```python
from build123d import *

# Parameters (mm, degrees)
SKETCH1_R                = 19.5
OUTERDIAMETERSTOCK_DEPTH = 115
SCREWONBASE_START        = -115
SCREWONBASE_DEPTH        = 5
INNERDIAMETER_START      = -3
SKETCH2_R                = 16
INNERDIAMETER_DEPTH      = 113
SKETCH3_R                = 10
HOLE_DEPTH               = 116
CUT_EXTRUDE3_REACH       = 117
SKETCH5_R                = 1.25
CHAMFER1_SIZE            = 1.5
WIRESLOT_START           = -115
SKETCH6_W                = 50
SKETCH6_H                = 20
WIRESLOT_DEPTH           = 10
MOUNTING_START           = -115
SKETCH7_R                = 2.5
MOUNTING_HOLES_DEPTH     = 5


with BuildPart() as part:
    # Sketch1 → OuterDiameterStock (new body)
    with BuildSketch(Plane(origin=(0, 0, 0), x_dir=(1, 0, 0), z_dir=(0, 1, 0))):
        Circle(SKETCH1_R)
    extrude(amount=-OUTERDIAMETERSTOCK_DEPTH)

    # Sketch4 → ScrewOnBase (add)
    with BuildSketch(Plane(origin=(0, 0, 0), x_dir=(1, 0, 0), z_dir=(0, 1, 0)).offset(SCREWONBASE_START)):
        with BuildLine():
            Line((0, 22.5), (50, 22.5))
            Line((50, 22.5), (50, -22.5))
            Line((50, -22.5), (0, -22.5))
            ThreePointArc((0, -22.5), (-22.5, 0), (0, 22.5))
        make_face()
    extrude(amount=SCREWONBASE_DEPTH)

    # Sketch2 → InnerDiameter (cut, through all)
    with BuildSketch(Plane(origin=(0, 0, 0), x_dir=(1, 0, 0), z_dir=(0, 1, 0)).offset(INNERDIAMETER_START)):
        Circle(SKETCH2_R)
    extrude(amount=-INNERDIAMETER_DEPTH, mode=Mode.SUBTRACT)

    # Sketch3 → Hole (cut, through all)
    with BuildSketch(Plane(origin=(0, 0, 0), x_dir=(1, 0, 0), z_dir=(0, 1, 0))):
        Circle(SKETCH3_R)
    extrude(amount=-HOLE_DEPTH, mode=Mode.SUBTRACT)

    # Sketch5 → Cut-Extrude3 (cut, up to next)
    with BuildSketch(Plane(origin=(0, 0, 0), x_dir=(1, 0, 0), z_dir=(0, 1, 0)), mode=Mode.PRIVATE) as cut_extrude3_sk1:
        with Locations((0, 13)):
            Circle(SKETCH5_R)
    cut_extrude3_tool1 = extrude(cut_extrude3_sk1.sketch, amount=-CUT_EXTRUDE3_REACH, mode=Mode.PRIVATE) & part.part
    add(cut_extrude3_tool1.solids().sort_by_distance((0, 0, -13))[0], mode=Mode.SUBTRACT)
    # Sketch5 → Cut-Extrude3 (cut, up to next)
    with BuildSketch(Plane(origin=(0, 0, 0), x_dir=(1, 0, 0), z_dir=(0, 1, 0)), mode=Mode.PRIVATE) as cut_extrude3_sk2:
        with Locations((13, 0)):
            Circle(SKETCH5_R)
    cut_extrude3_tool2 = extrude(cut_extrude3_sk2.sketch, amount=-CUT_EXTRUDE3_REACH, mode=Mode.PRIVATE) & part.part
    add(cut_extrude3_tool2.solids().sort_by_distance((13, 0, 0))[0], mode=Mode.SUBTRACT)
    # Sketch5 → Cut-Extrude3 (cut, up to next)
    with BuildSketch(Plane(origin=(0, 0, 0), x_dir=(1, 0, 0), z_dir=(0, 1, 0)), mode=Mode.PRIVATE) as cut_extrude3_sk3:
        with Locations((0, -13)):
            Circle(SKETCH5_R)
    cut_extrude3_tool3 = extrude(cut_extrude3_sk3.sketch, amount=-CUT_EXTRUDE3_REACH, mode=Mode.PRIVATE) & part.part
    add(cut_extrude3_tool3.solids().sort_by_distance((0, 0, 13))[0], mode=Mode.SUBTRACT)
    # Sketch5 → Cut-Extrude3 (cut, up to next)
    with BuildSketch(Plane(origin=(0, 0, 0), x_dir=(1, 0, 0), z_dir=(0, 1, 0)), mode=Mode.PRIVATE) as cut_extrude3_sk4:
        with Locations((-13, 0)):
            Circle(SKETCH5_R)
    cut_extrude3_tool4 = extrude(cut_extrude3_sk4.sketch, amount=-CUT_EXTRUDE3_REACH, mode=Mode.PRIVATE) & part.part
    add(cut_extrude3_tool4.solids().sort_by_distance((-13, 0, 0))[0], mode=Mode.SUBTRACT)

    # Chamfer1
    chamfer1_edges = [part.edges().sort_by_distance(p)[0] for p in [
        (-1.25, 0, -13),
        (11.75, 0, 0),
        (-1.25, 0, 13),
        (-14.25, 0, 0),
    ]]
    chamfer(chamfer1_edges, length=CHAMFER1_SIZE)

    # Sketch6 → WireSlot (cut)
    with BuildSketch(Plane(origin=(0, 0, 0), x_dir=(1, 0, 0), z_dir=(0, 1, 0)).offset(WIRESLOT_START)):
        with Locations((25, 0)):
            Rectangle(SKETCH6_W, SKETCH6_H)
    extrude(amount=WIRESLOT_DEPTH, mode=Mode.SUBTRACT)

    # Sketch7 → Mounting Holes (cut)
    with BuildSketch(Plane(origin=(0, 0, 0), x_dir=(1, 0, 0), z_dir=(0, 1, 0)).offset(MOUNTING_START)):
        with Locations((30, 16.25)):
            Circle(SKETCH7_R)
        with Locations((30, -16.25)):
            Circle(SKETCH7_R)
    extrude(amount=MOUNTING_HOLES_DEPTH, mode=Mode.SUBTRACT)


solid = part.part
```
CAD build for the part. Positions are in the model's coordinates, mm. A direction names the side the tool comes from. Round coordinates to 2 decimals unless told otherwise and drop trailing zeros. Loops run counter-clockwise (first coordinate to the right, second up) from the corner with the lowest first, then second, coordinate; pieces in that order, holes last. Notation, with made-up numbers: M -21,14 L 29,14 A13 ccw 29,35 Z; hole C 19,44.25 d3. An arc over 180 degrees is marked long. Return JSON: item names as keys, results as strings. Group by question number.
(1) Saw through at B-B, the plane y = -15. List the corners of the cut face in (x, z).
(2) Saw through at D-D, the plane x = -13. List the corners of the cut face in (y, z).
(3) Tool access for faces 1 (the cylindrical face through (-15.985, -58.216, -0.703)), 2 (the flat face through (-9, 0, -5)), 3 (the flat face through (17, -105, 0)): list every direction of +Z, -Z, +X, -X, +Y, -Y with a clear straight run to the whole face (end or side of a thin tool).
(4) Drop flat-ended pins along their axis: P1, Ø3, axis at x = 0, z = 13, coming from the -Y side; P2, Ø1.5, axis at x = 37.5, z = 16.5, coming from the +Y side; P3, Ø11, axis at x = 28, y = -109.5, coming from the +Z side; P4, Ø6, axis at x = -13.5, y = -18.5, coming from the -Z side. Give the stop position or say it passes through.
(5) Saw through at A-A, the plane x = 34.5. List the corners of the cut face in (y, z).
(6) Saw through at C-C, the plane z = 8. List the corners of the cut face in (x, y), and give its area (3 significant figures).
(7) Mould opens along Z. For faces 4 (the flat face through (25, -113, -22.5)), 5 (the flat face through (31, -112, -10)), 6 (the flat face through (50, -113, -16)) say: +Z half, -Z half, draft (parallel to the pull), parting line (faces both ways), or undercut.
(8) Wall check: probe 1 along Z at (x, y) = (30, -112.6); probe 2 along Z at (x, y) = (0, -1.9); probe 3 along X at (y, z) = (-73, 0). Give the ranges that are in metal, low to high. Write a range as [from, to].
Answer list:
{
 "1": {"outline": "C 0,0 d39; hole C 0,0 d32"},
 "2": {"outline": "M -115,-18.36 L -110,-18.36 L -110,-14.53 L 0,-14.53 L 0,-2.75 L -1.5,-1.25 L -3,-1.25 L -3,-9.33 L -115,-9.33 Z; M -115,9.33 L -3,9.33 L -3,1.25 L -1.5,1.25 L 0,2.75 L 0,14.53 L -110,14.53 L -110,18.36 L -115,18.36 Z"},
 "3": {"face 1": "-Y", "face 2": "+Z, -Z, +X, -X, +Y", "face 3": "+X, -Y"},
 "4": {"P1": "y = -3", "P2": "y = -110", "P3": "z = 22.5", "P4": "z = -16.43"},
 "5": {"outline": "M -115,-22.5 L -110,-22.5 L -110,-10 L -115,-10 Z; M -115,10 L -110,10 L -110,22.5 L -115,22.5 Z"},
 "6": {"outline": "M -21.03,-115 L -13.86,-115 L -13.86,-3 L -6,-3 L -6,0 L -17.78,0 L -17.78,-110 L -21.03,-110 Z; M 6,-3 L 13.86,-3 L 13.86,-105 L 17.78,-105 L 17.78,0 L 6,0 Z", "area": "927 mm2"},
 "7": {"face 4": "-Z half", "face 5": "undercut", "face 6": "draft"},
 "8": {"probe 1": "[-22.5, -18.75], [-13.75, -10], [10, 13.75], [18.75, 22.5]", "probe 2": "[-19.5, -14.25], [-11.75, -10], [10, 11.75], [14.25, 19.5]", "probe 3": "[-19.5, -16], [16, 19.5]"}
}
